from build123d import *

# Parameters (mm, degrees)
F0_R     = 45
F0_R_2   = 35
F1_DEPTH = 3
F2_R     = 1.9
F3_DEPTH = 25
F4_W     = 55.17469
F4_H     = 97.550949
F5_DEPTH = 25


with BuildPart() as f1:
    # F0 (on Top) → F1 (new body)
    with BuildSketch(Plane.XY):
        Circle(F0_R)
        Circle(F0_R_2, mode=Mode.SUBTRACT)
    extrude(amount=F1_DEPTH)

    # F2 (on face) → F3 (cut)
    with BuildSketch(Plane.XY.offset(3)):
        with Locations((-40, 0)):
            Circle(F2_R)
        with Locations((40, 0)):
            Circle(F2_R)
    extrude(amount=-F3_DEPTH, mode=Mode.SUBTRACT)

    # F4 (on face) → F5 (cut)
    with BuildSketch(Plane.XY.offset(3)):
        with Locations((27.587345, 3.775474)):
            Rectangle(F4_W, F4_H)
    extrude(amount=-F5_DEPTH, mode=Mode.SUBTRACT)

    # F6: F1 across face


with BuildPart() as f1_1:
    add(f1.part)
    add(f1.part.mirror(Plane(origin=(0, 40, 1.5), x_dir=(0, 1, 0), z_dir=(1, 0, 0))))


solid = f1_1.part
CAD build for the part. Positions are in the model's coordinates, mm. Round coordinates to 2 decimals unless told otherwise and drop trailing zeros. Write each loop counter-clockwise with the first axis right and the second up, starting at its lowest first coordinate (ties: lowest second). Pieces come first, ordered by that corner, then holes. Notation, with made-up numbers: M 21.5,57 L 64.5,57 A15 cw 64.5,64 Z; hole C -11.75,-24 d10. An arc over 180 degrees is marked long. Put each result on its own line as item: value. Start each with the question number.
1) Saw through at C-C, the plane y = 9.5. Write the cut outline in (x, z).
2) Saw through at A-A, the plane y = 0. Write the cut outline in (x, z).
3) Pin check, flat tips, straight feed: pin 1 Ø1.5 at (x, z) = (20.5, 1) entering from +Y; pin 2 Ø1.5 at (x, z) = (-7.5, 2) entering from -Y; pin 3 Ø1 at (x, z) = (13.5, 1.5) entering from -Y. Stop position of each tip, or through.
4) Pull direction X, two halves, no side cores. Call faces 1 (the cylindrical face through (13.41, 32.33, 1.48)), 2 (the cylindrical face through (-17.235, 41.569, 1.479)), 3 (the cylindrical face through (-38.188, 0.571, 1.521)), 4 (the flat face through (-23.1, -26.5, 0)): pulls with the +X half, pulls with the -X half, needs draft (parallel to the pull), parting line crosses it, or undercut.
5) Drill centre lines: probe 1 along Y at (x, z) = (0, 1.6); probe 2 along X at (y, z) = (-26, 0.9); probe 3 along Y at (x, z) = (-7, 0.9). Where is each one in solid material? Low to high. Write a range as [from, to].
6) Saw through at D-D, the plane z = 0.55. Write the cut outline in (x, y), and give its area (3 significant figures).
7) Saw through at B-B, the plane x = 0. Write the cut outline in (y, z).
Resolved:
1. outline: M -43.99,0 L -33.69,0 L -33.69,3 L -43.99,3 Z; M 33.69,0 L 43.99,0 L 43.99,3 L 33.69,3 Z
2. outline: M -45,0 L -41.9,0 L -41.9,3 L -45,3 Z; M -38.1,0 L -35,0 L -35,3 L -38.1,3 Z; M 35,0 L 38.1,0 L 38.1,3 L 35,3 Z; M 41.9,0 L 45,0 L 45,3 L 41.9,3 Z
3. pin 1: y = 40.43
3. pin 2: y = -44.49
3. pin 3: y = -43.08
4. face 1: undercut
4. face 2: parting line crosses it
4. face 3: undercut
4. face 4: needs draft
5. probe 1: [-45, -35], [35, 45]
5. probe 2: [-36.73, -23.43], [23.43, 36.73]
5. probe 3: [-44.45, -34.29], [34.29, 44.45]
6. outline: C 0,0 d90; hole C -40,0 d3.8; hole C 0,0 d70; hole C 40,0 d3.8
6. area: 2,490 mm²
7. outline: M -45,0 L -35,0 L -35,3 L -45,3 Z; M 35,0 L 45,0 L 45,3 L 35,3 Z
